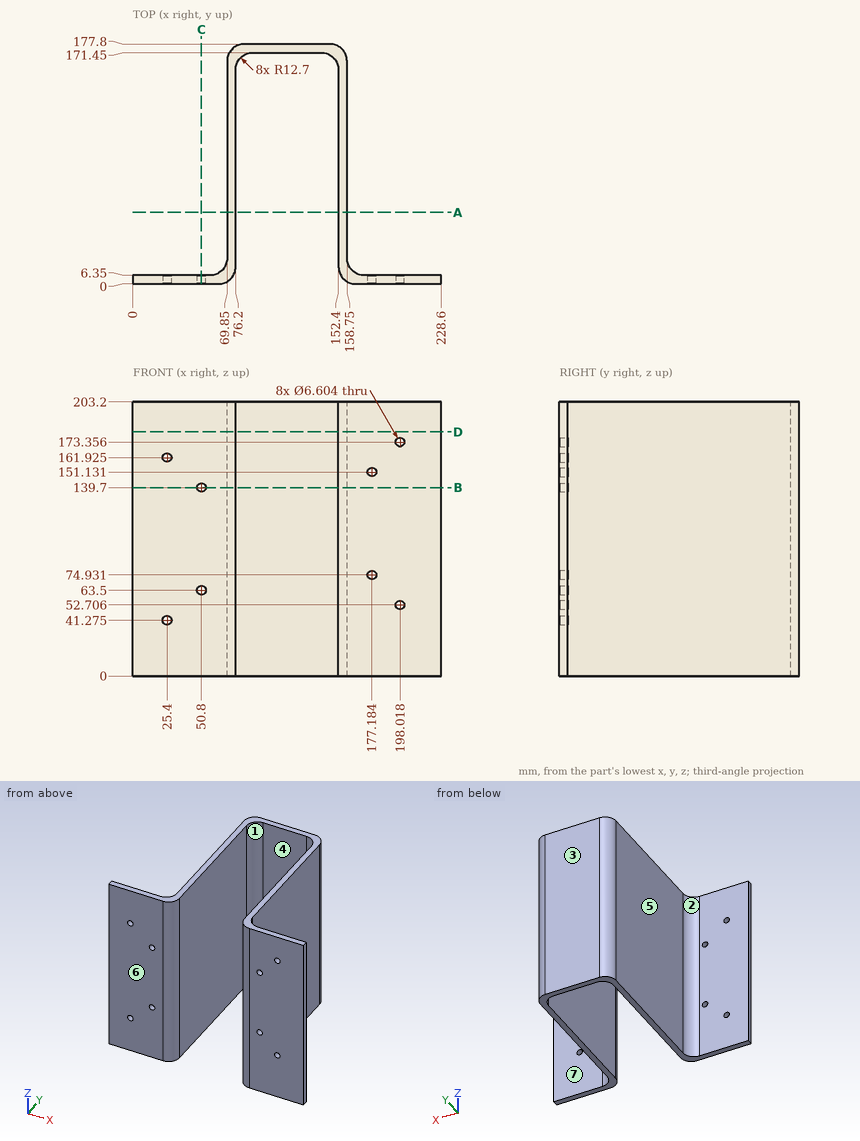
Drawing for the job (mm, zero at the part's lowest x, y, z). A direction names the side the tool comes from. Round coordinates to 2 decimals unless told otherwise and drop trailing zeros. Loops run counter-clockwise (first coordinate to the right, second up) from the corner with the lowest first, then second, coordinate; pieces in that order, holes last. Notation, with made-up numbers: (24.25, 75) -> (53.25, 75) arc R13 cw to (53.25, 79) -> close; hole circle Ø1 at (15, -33). An arc over 180 degrees is marked (long way). Answer in a Markdown table with one row per item.
Item 1: Drill centre lines: L1, parallel to Z at x = 50.8, y = 3.5; L2, parallel to Z at x = 25.4, y = 2; L3, parallel to X at y = 86, z = 134. Where is each one in solid material? Low to high. Write a range as [from, to].
Answers below:
| item | result |
|---|---|
| L1 | z = [0, 60.2], [66.8, 136.4], [143, 203.2] |
| L2 | z = [0, 37.97], [44.58, 158.62], [165.23, 203.2] |
| L3 | x = [69.85, 76.2], [152.4, 158.75] |
Item 2: Which spindle directions (+Z, -Z, +X, -X, +Y, -Y) get a long thin tool onto all of the face, cutting with end or side? Do the marked faces 4, 5, 6 and 7. Say none if no direction does.
Answers below:
| item | result |
|---|---|
| face 4 | +Z, -Z, -Y |
| face 5 | +Z, -Z, -X, +Y |
| face 6 | +Z, -Z, +X, -X, -Y |
| face 7 | +Z, -Z, +X, +Y |
Item 3: Pin check, flat tips, straight feed: pin 1 (2 mm diameter, centred on x = 203.5, z = 161.5, fed in from +Y); pin 2 (8.5 mm diameter, centred on x = 50.8, z = 139.7, fed in from -Y); pin 3 (12 mm diameter, centred on y = 157, z = 69, fed in from +X); pin 4 (4 mm diameter, centred on x = 198.02, z = 52.71, fed in from +Y). Stop position of each tip, or through.
Answers below:
| item | result |
|---|---|
| pin 1 | stops at y = 6.35 |
| pin 2 | stops at y = 0 |
| pin 3 | stops at x = 158.75 |
| pin 4 | passes through |
Item 4: Saw through at A-A (y = 53). Write the cut outline in (x, z).
Answers below:
| item | result |
|---|---|
| outline | (69.85, 0) -> (76.2, 0) -> (76.2, 203.2) -> (69.85, 203.2) -> close; (152.4, 0) -> (158.75, 0) -> (158.75, 203.2) -> (152.4, 203.2) -> close |
Item 5: Saw through at C-C (x = 50.8). Write the cut outline in (y, z).
Answers below:
| item | result |
|---|---|
| outline | (0, 0) -> (6.35, 0) -> (6.35, 60.2) -> (0, 60.2) -> close; (0, 66.8) -> (6.35, 66.8) -> (6.35, 136.4) -> (0, 136.4) -> close; (0, 143) -> (6.35, 143) -> (6.35, 203.2) -> (0, 203.2) -> close |
Item 6: Saw through at B-B (z = 139.7). Write the cut outline in (x, y), and give its area (3 significant figures).
Answers below:
| item | result |
|---|---|
| outline | (0, 0) -> (47.5, 0) -> (47.5, 6.35) -> (0, 6.35) -> close; (54.1, 0) -> (63.5, 0) arc R12.7 ccw to (76.2, 12.7) -> (76.2, 158.75) arc R12.7 cw to (88.9, 171.45) -> (139.7, 171.45) arc R12.7 cw to (152.4, 158.75) -> (152.4, 12.7) arc R12.7 ccw to (165.1, 0) -> (228.6, 0) -> (228.6, 6.35) -> (171.45, 6.35) arc R12.7 cw to (158.75, 19.05) -> (158.75, 165.1) arc R12.7 ccw to (146.05, 177.8) -> (82.55, 177.8) arc R12.7 ccw to (69.85, 165.1) -> (69.85, 19.05) arc R12.7 cw to (57.15, 6.35) -> (54.1, 6.35) -> close |
| area | 3,590 mm² |
Item 7: Mould opens along X. For the marked faces 1, 2 and 3 say: +X half, -X half, draft (parallel to the pull), parting line (faces both ways), or undercut.
Answers below:
| item | result |
|---|---|
| face 1 | undercut |
| face 2 | -X half |
| face 3 | draft |
Item 8: Saw through at D-D (z = 181). Write the cut outline in (x, y).
Answers below:
| item | result |
|---|---|
| outline | (0, 0) -> (63.5, 0) arc R12.7 ccw to (76.2, 12.7) -> (76.2, 158.75) arc R12.7 cw to (88.9, 171.45) -> (139.7, 171.45) arc R12.7 cw to (152.4, 158.75) -> (152.4, 12.7) arc R12.7 ccw to (165.1, 0) -> (228.6, 0) -> (228.6, 6.35) -> (171.45, 6.35) arc R12.7 cw to (158.75, 19.05) -> (158.75, 165.1) arc R12.7 ccw to (146.05, 177.8) -> (82.55, 177.8) arc R12.7 ccw to (69.85, 165.1) -> (69.85, 19.05) arc R12.7 cw to (57.15, 6.35) -> (0, 6.35) -> close |
